Autodesk Inventor part; units mm, degrees
ref_plane "YZ Plane" through (0, 0, 0) normal (1, 0, 0) x (0, 1, 0)
ref_plane "XZ Plane" through (0, 0, 0) normal (0, 1, 0) x (-1, 0, 0)
ref_plane "XY Plane" through (0, 0, 0) normal (0, 0, 1) x (1, 0, 0)
sketch "Sketch1" plane through (0, 0, 0) normal (0, 0, 1) x (1, 0, 0)
  line L0 (3, -6.7347) -> (-5, -6.7347)
  line L1 (-5, -6.7347) -> (-5, 3.2653)
  line L2 (-1, 7.2653) -> (-1, 7.2653)
  line L3 (3, 3.2653) -> (3, -6.7347)
  arc A0 (3, 3.2653) -> (-1, 7.2653) centre (-1, 3.2653) ccw
  arc A1 (-1, 7.2653) -> (-5, 3.2653) centre (-1, 3.2653) ccw
  point P0 (0, 0)
  point P1 (-5, 7.2653)
  point P2 (3, 7.2653)
  point P3 (-1, 7.2653)
  dimension "d0" = 8
  dimension "d1" = 14
  dimension "d2" = 4
revolve "Revolution1" add sketch "Sketch1" angle 360 about axis through (3, 3.2653, 0) along (0, -1, 0)
sketch "Sketch2" plane through (3, -6.7347, 0) normal (0, -1, 0) x (1, 0, 0)
  circle A0 centre (0, 2.4175) radius 0.5
  circle A1 centre (0, -2.4175) radius 0.5
  point P0 (-3, 0)
  dimension "d4" = 1
  dimension "d5" = 1
  dimension "d8" = 4.8351
sketch "Sketch3" plane through (3, -6.7347, 0) normal (0, -1, 0) x (1, 0, 0)
  point P0 (-3, 0)
extrude "Extrusion1" add sketch "Sketch2" along normal blind 10
properties part number "LED"
Work out the finished part from the listing and answer in its coordinate system (mm). A direction names the side the tool comes from. Round coordinates to 2 decimals unless told otherwise and drop trailing zeros. Write each loop counter-clockwise with the first axis right and the second up, starting at its lowest first coordinate (ties: lowest second). Pieces come first, ordered by that corner, then holes. Notation, with made-up numbers: (4, 65.25) - (63, 65.25) arc R37 cw to (63, 101.25) - close; hole circle Ø3 at (59.25, -2). An arc over 180 degrees is marked (long way). Return JSON: item names as keys, results as strings. Group by question number.
Q1. For faces 1 (the cylindrical face through (2.603, -11.665, -2.113)), 2 (the flat face through (3, -16.735, 2.4)), determine the directions among +Z, -Z, +X, -X, +Y, -Y from which every point of the face is accessible in a straight line to the end or side of a thin tool.
Q2. Find the intervals of material crossed by L1, parallel to Y at x = 0.75, z = 1.25; L2, parallel to Y at x = 4.75, z = 7.25; L3, parallel to X at y = 4.5, z = -3, in increasing order.
Q3. The mould has two halves that part along Z. Classify faces 3 (the flat face through (3, -16.735, -2.4)), 4 (the cylindrical face through (2.5, -11.7, 2.4)), 5 (the cylindrical face through (4.73, -1.66, -7.81)): released by +Z, released by -Z, zero draft, split by the parting line, or undercut.
Q4. Each of these flat-tipped pins is pushed along its axis until it touches: pin 1 Ø4 at (y, z) = (-9.5, 2.5) entering from -X; pin 2 Ø3 at (y, z) = (-14, -3.5) entering from +X; pin 3 Ø1 at (x, z) = (1, -1.5) entering from +Y. Where does it stop, or does it pass through?
Q5. The part is cut by section B-B on y = -2.5. Write down the section's boundary in (x, z), then the cut area to 3 significant figures.
Q6. The part is cut by section A-A on y = -9. Write down the section's boundary in (x, z).
Solved:
{
 "1": {"face 1": "-Y", "face 2": "+Z, -Z, +X, -X, -Y"},
 "2": {"L1": "-6.73 to 7", "L2": "-6.73 to 5.28", "L3": "-4.21 to 10.21"},
 "3": {"face 3": "zero draft", "face 4": "undercut", "face 5": "split by the parting line"},
 "4": {"pin 1": "x = 2.5", "pin 2": "x = 3.5", "pin 3": "y = 7.14"},
 "5": {"outline": "circle Ø16 at (3, 0)", "area": "201 mm²"},
 "6": {"outline": "circle Ø1 at (3, -2.42); circle Ø1 at (3, 2.42)"}
}
